Input: part model. Units: mm. Frame: model coordinates. A direction names the side the tool comes from. Give positions to 0.01 mm unless a question says otherwise; leave off trailing zeros. Loops run counter-clockwise (first coordinate to the right, second up) from the corner with the lowest first, then second, coordinate; pieces in that order, holes last. Notation, with made-up numbers: M 17.5,49.25 L 41.5,49.25 A17 cw 41.5,60.25 Z; hole C 29,-26.75 d2. An arc over 180 degrees is marked long. Answer as a JSON object with one key per item and string values. Group by question number.
1) Draft query along X for faces 1 (the cylindrical face through (-58.426, -27.727, 9.569)), 2 (the flat face through (11.112, 78, 6)), 3 (the flat face through (-1, 1, 12.7)). Return one class per face: +X half, -X half, draft (parallel to the pull), parting line (faces both ways), or undercut.
2) Section query D-D on x = -21.5. Return loops of the section in (y, z).
3) First-contact query: P1, Ø1.6, axis at y = 0, z = 6.35, coming from the -X side; P2, Ø3, axis at y = -78.5, z = 7.5, coming from the -X side; P3, Ø3, axis at x = 64.5, z = 6, coming from the +Y side. Flat tips, straight axial feed; report the tip coordinate or a pass-through.
4) Section query A-A on x = 0. Return loops of the section in (y, z).
5) Section query C-C on z = 9.75. Count the separate pieces of the cut face and the enclosed holes in it, plus the area to 3 significant figures.
6) Section query B-B on y = -38. Return loops of the section in (x, z), plus the area to 3 significant figures.
7) Access query for faces 4 (the flat face through (0, -76.2, 6)), 5 (the flat face through (-65, -57, 6.35)), 6 (the flat face through (-82.55, -1, 8)). Directions: +Z, -Z, +X, -X, +Y, -Y. A direction counts if a zero-diameter tool reaches every point of the face in a straight line with its end or side. Return the directions, or none.
8) Ray query, L1, parallel to X at y = -50.5, z = 5.75; L2, parallel to X at y = -32.5, z = 10.5; L3, parallel to Y at x = -50.8, z = 4. Return the intervals inside material, ascending.
from build123d import *

# Parameters (mm, degrees)
SKETCH1_W             = 165.1
SKETCH1_H             = 152.4
BOSS_EXTRUDE1_DEPTH   = 12.7
BOSS_EXTRUDE2_DEPTH   = 12.7
CUT_EXTRUDE1_REACH    = 119.432
BOSS_EXTRUDE3_DEPTH   = 12.7
CUT_EXTRUDE2_DEPTH    = 12.7
SKETCH7_R             = 11.1125
CUT_EXTRUDE3_DEPTH    = 12.7
M3_CLEARANCE_HOLE1_D  = 3.4
SKETCH14_R            = 4.7625
CUT_EXTRUDE5_DEPTH    = 6.35
SKETCH13_R            = 3.175
CUT_EXTRUDE7_DEPTH    = 6.35
F_8_CLEARANCE_HOLE1_D = 4.4958
SKETCH18_R            = 5.08
CUT_EXTRUDE8_DEPTH    = 6.35
SKETCH20_R            = 0.99187
CUT_EXTRUDE9_DEPTH    = 25.4


with BuildPart() as part:
    # Sketch1 → Boss-Extrude1 (new body)
    with BuildSketch(Plane.XY):
        Rectangle(SKETCH1_W, SKETCH1_H)
    extrude(amount=BOSS_EXTRUDE1_DEPTH)

    # Sketch2 → Boss-Extrude2 (add)
    with BuildSketch(Plane.XY.offset(12.7)):
        Polygon((-11.1125, 76.2), (11.1125, 76.2), (11.1125, 80.01), (10.664629469, 82.55), (-10.664629469, 82.55), (-11.1125, 80.01), align=None)
    extrude(amount=-BOSS_EXTRUDE2_DEPTH)

    # Sketch4 → Cut-Extrude1 (cut, up to next)
    with BuildSketch(Plane.XY.offset(12.7), mode=Mode.PRIVATE) as cut_extrude1_sk1:
        with BuildLine():
            Line((-17.7165, 76.2), (-11.1125, 76.2))
            ThreePointArc((-11.1125, 76.2), (-14.4145, 72.898), (-17.7165, 76.2))
        make_face()
    cut_extrude1_tool1 = extrude(cut_extrude1_sk1.sketch, amount=-CUT_EXTRUDE1_REACH, mode=Mode.PRIVATE) & part.part
    # Sketch4 → Cut-Extrude1 (cut, up to next)
    with BuildSketch(Plane.XY.offset(12.7), mode=Mode.PRIVATE) as cut_extrude1_sk2:
        with BuildLine():
            Line((11.1125, 76.2), (17.7165, 76.2))
            ThreePointArc((17.7165, 76.2), (14.4145, 72.898), (11.1125, 76.2))
        make_face()
    cut_extrude1_tool2 = extrude(cut_extrude1_sk2.sketch, amount=-CUT_EXTRUDE1_REACH, mode=Mode.PRIVATE) & part.part
    add(cut_extrude1_tool1.solids().sort_by_distance((-14.4145, 74.798588, 12.7))[0], mode=Mode.SUBTRACT)
    add(cut_extrude1_tool2.solids().sort_by_distance((14.4145, 74.798588, 12.7))[0], mode=Mode.SUBTRACT)

    # Sketch5 → Boss-Extrude3 (add)
    with BuildSketch(Plane.XY.offset(12.7)):
        Polygon((63.5, -76.2), (41.275, -76.2), (41.275, -80.01), (41.722870531, -82.55), (63.052129469, -82.55), (63.5, -80.01), align=None)
    boss_extrude3 = extrude(amount=-BOSS_EXTRUDE3_DEPTH)

    # Sketch6 → Cut-Extrude2 (cut)
    with BuildSketch(Plane.XY.offset(12.7)):
        with BuildLine():
            Line((34.671, -76.2), (41.275, -76.2))
            ThreePointArc((41.275, -76.2), (37.973, -72.898), (34.671, -76.2))
        make_face()
        with BuildLine():
            Line((63.5, -76.2), (70.104, -76.2))
            ThreePointArc((70.104, -76.2), (66.802, -72.898), (63.5, -76.2))
        make_face()
    cut_extrude2 = extrude(amount=-CUT_EXTRUDE2_DEPTH, mode=Mode.SUBTRACT)

    # Mirror1: Boss-Extrude3, Cut-Extrude2 across plane
    add(boss_extrude3.mirror(Plane(origin=(0, 0, 0), x_dir=(0, 0, 1), z_dir=(1, 0, 0))))
    add(cut_extrude2.mirror(Plane(origin=(0, 0, 0), x_dir=(0, 0, 1), z_dir=(1, 0, 0))), mode=Mode.SUBTRACT)

    # Sketch7 → Cut-Extrude3 (cut)
    with BuildSketch(Plane.XY.offset(12.7)):
        with Locations((-47.625, -41.275)):
            Circle(SKETCH7_R)
        with Locations((47.625, -41.275)):
            Circle(SKETCH7_R)
    extrude(amount=-CUT_EXTRUDE3_DEPTH, mode=Mode.SUBTRACT)

    # M3 Clearance Hole1 (through all)
    with Locations(Plane.XY.offset(12.7)):
        with Locations((-63.119, -25.781), (-32.131, -25.781), (-32.131, -56.769), (-63.119, -56.769)):
            m3_clearance_hole1 = Hole(M3_CLEARANCE_HOLE1_D / 2)

    # Mirror2: M3 Clearance Hole1 across plane
    add(m3_clearance_hole1.mirror(Plane(origin=(0, 0, 0), x_dir=(0, 0, 1), z_dir=(1, 0, 0))), mode=Mode.SUBTRACT)

    # Sketch14 → Cut-Extrude5 (cut)
    with BuildSketch(Plane.XY.offset(12.7)):
        with Locations((-50.8, 30.528732114)):
            Circle(SKETCH14_R)
        with Locations((63.5, 30.528732114)):
            Circle(SKETCH14_R)
    extrude(amount=-CUT_EXTRUDE5_DEPTH, mode=Mode.SUBTRACT)

    # Sketch13 → Cut-Extrude7 (cut)
    with BuildSketch(Plane.XY.offset(12.7)):
        with Locations((0, -12.655936751)):
            Circle(SKETCH13_R)
    extrude(amount=-CUT_EXTRUDE7_DEPTH, mode=Mode.SUBTRACT)

    # #8 Clearance Hole1 (through all)
    with Locations(Plane.XY.offset(12.7)):
        with Locations((0, -12.655936751), (63.5, 30.528732114), (-50.8, 30.528732114)):
            Hole(F_8_CLEARANCE_HOLE1_D / 2)

    # Sketch18 → Cut-Extrude8 (cut)
    with BuildSketch(Plane.XY.offset(12.7)):
        with Locations((-63.119, -25.781)):
            Circle(SKETCH18_R)
        with Locations(Location((-63.119, -56.769, 0), (0, 0, 180))):
            Circle(SKETCH18_R)
        with Locations((-32.131, -56.769)):
            Circle(SKETCH18_R)
        with Locations(Location((-32.131, -25.781, 0), (0, 0, 180))):
            Circle(SKETCH18_R)
        with Locations((32.131, -25.781)):
            Circle(SKETCH18_R)
        with Locations(Location((32.131, -56.769, 0), (0, 0, 180))):
            Circle(SKETCH18_R)
        with Locations((63.119, -56.769)):
            Circle(SKETCH18_R)
        with Locations(Location((63.119, -25.781, 0), (0, 0, 180))):
            Circle(SKETCH18_R)
    extrude(amount=-CUT_EXTRUDE8_DEPTH, mode=Mode.SUBTRACT)

    # Sketch20 → Cut-Extrude9 (cut)
    with BuildSketch(Plane(origin=(82.55, 0, 0), x_dir=(0, 0, -1), z_dir=(1, 0, 0))):
        with Locations((-6.35, 0)):
            Circle(SKETCH20_R)
    cut_extrude9 = extrude(amount=-CUT_EXTRUDE9_DEPTH, mode=Mode.SUBTRACT)

    # Mirror3: Cut-Extrude9 across plane
    add(cut_extrude9.mirror(Plane(origin=(0, 0, 0), x_dir=(0, 0, 1), z_dir=(1, 0, 0))), mode=Mode.SUBTRACT)


solid = part.part
Output:
{
 "1": {"face 1": "undercut", "face 2": "+X half", "face 3": "draft"},
 "2": {"outline": "M -76.2,0 L 76.2,0 L 76.2,12.7 L -76.2,12.7 Z"},
 "3": {"P1": "stops at x = -57.15", "P2": "stops at x = -63.5", "P3": "stops at y = 76.2"},
 "4": {"outline": "M -76.2,0 L -14.9,0 L -14.9,6.35 L -15.83,6.35 L -15.83,12.7 L -76.2,12.7 Z; M -10.41,0 L 82.55,0 L 82.55,12.7 L -9.48,12.7 L -9.48,6.35 L -10.41,6.35 Z"},
 "5": {"separate pieces": "1", "enclosed holes": "13", "area": "23,900 mm^2"},
 "6": {"outline": "M -82.55,0 L -58.24,0 L -58.24,12.7 L -82.55,12.7 Z; M -37.01,0 L 37.01,0 L 37.01,12.7 L -37.01,12.7 Z; M 58.24,0 L 82.55,0 L 82.55,12.7 L 58.24,12.7 Z", "area": "1,560 mm^2"},
 "7": {"face 4": "+Z, -Z, -Y", "face 5": "+Z", "face 6": "+Z, -Z, -X, +Y, -Y"},
 "8": {"L1": "x = -82.55 to -53.82, -41.43 to 41.43, 53.82 to 82.55", "L2": "x = -82.55 to -54.44, -40.81 to 40.81, 54.44 to 82.55", "L3": "y = -82.55 to -51.92, -30.63 to 28.28, 32.78 to 76.2"}
}
